Can you work these out from the model? Positions are in its coordinate system, mm. A direction names the side the tool comes from. Coordinates: 2 decimals unless noted, no trailing zeros. Order: outer loops, then holes, each group sorted by start corner. A loop starts at its lowest first (then second) coordinate and runs counter-clockwise, first axis right, second up. Notation, with made-up numbers: (18.5, 58.25) -> (64.5, 58.25) arc R29 cw to (64.5, 90.25) -> close; hole circle Ø10 at (9.25, -12.5). An arc over 180 degrees is marked (long way). Use a Markdown table: item, result. Add a question column.
1. For faces 1 (the cylindrical face through (0, 2, 9)), 2 (the cylindrical face through (3, 2, 6)), 3 (the cylindrical face through (0, 2, 3)), 4 (the cylindrical face through (-3, 2, 6)), which set-ups out of +Z, -Z, +X, -X, +Y, -Y let a thin tool reach every point of the face, with its end or its side?
2. Suppose I cut it at A-A, the plane y = 0. List the corners of the cut face in (x, z) for me, then the cut area to 3 significant figures.
3. Suppose I cut it at C-C, the plane z = 8.5. List the corners of the cut face in (x, y) for me.
4. Suppose I cut it at B-B, the plane x = -2.5. List the corners of the cut face in (y, z) for me.
5. If I drill on line 1 along X through (y, z) = (0, 2); line 2 along Z through (x, y) = (3, -1.15); line 3 along Y through (x, z) = (1.5, 2.75), over which ranges is the centre line in solid material (lowest first)? Write a range as from..to.
6. For pin 1 Ø1.5 at (x, z) = (4, 7) entering from -Y; pin 2 Ø1 at (x, y) = (4, -0.5) entering from +Z; pin 3 Ø1 at (x, y) = (2, 0.5) entering from +Z; pin 4 Ø1.5 at (x, z) = (2.5, 5.5) entering from +Y, each with a flat end and sliding along its axis, tell me the tip position at first contact or that it passes through.
```python
from build123d import *

# Parameters (mm, degrees)
SKETCH1_R           = 2
BOSS_EXTRUDE1_DEPTH = 12
SKETCH3_R           = 2
BOSS_EXTRUDE2_DEPTH = 6
CHAMFER1_SIZE       = 0.5
CHAMFER2_SIZE       = 0.5


with BuildPart() as part:
    # Sketch1 → Boss-Extrude1 (new body)
    with BuildSketch(Plane.XY):
        Circle(SKETCH1_R)
    extrude(amount=BOSS_EXTRUDE1_DEPTH)

    # Sketch3 → Boss-Extrude2 (add, symmetric)
    with BuildSketch(Plane(origin=(0, 0, 0), x_dir=(0, 0, -1), z_dir=(1, 0, 0))):
        with Locations(Location((-6, 0, 0), (0, 0, 270))):
            Circle(SKETCH3_R)
    extrude(amount=BOSS_EXTRUDE2_DEPTH, both=True)

    # Chamfer1
    chamfer1_edges = [part.edges().sort_by_distance(p)[0] for p in [
        (6, 2, 6),
    ]]
    chamfer(chamfer1_edges, length=CHAMFER1_SIZE)

    # Chamfer2
    chamfer2_edges = [part.edges().sort_by_distance(p)[0] for p in [
        (-2, 0, 0),
        (-2, 0, 12),
        (-6, 2, 6),
    ]]
    chamfer(chamfer2_edges, length=CHAMFER2_SIZE)


solid = part.part
```
Worked out:
| question | item | result |
|---|---|---|
| 1 | face 1 | +Z |
| 1 | face 2 | +X |
| 1 | face 3 | -Z |
| 1 | face 4 | -X |
| 2 | outline | (-6, 4.5) -> (-5.5, 4) -> (-2, 4) -> (-2, 0.5) -> (-1.5, 0) -> (1.5, 0) -> (2, 0.5) -> (2, 4) -> (5.5, 4) -> (6, 4.5) -> (6, 7.5) -> (5.5, 8) -> (2, 8) -> (2, 11.5) -> (1.5, 12) -> (-1.5, 12) -> (-2, 11.5) -> (-2, 8) -> (-5.5, 8) -> (-6, 7.5) -> close |
| 2 | area | 79.0 mm² |
| 3 | outline | circle Ø4 at (0, 0) |
| 4 | outline | circle Ø4 at (0, 6) |
| 5 | line 1 | x = -2..2 |
| 5 | line 2 | z = 4.36..7.64 |
| 5 | line 3 | y = -1.32..1.32 |
| 6 | pin 1 | stops at y = -1.98 |
| 6 | pin 2 | stops at z = 8 |
| 6 | pin 3 | stops at z = 11.94 |
| 6 | pin 4 | stops at y = 2 |
